CAD build for the part. Positions are in the model's coordinates, mm. A direction names the side the tool comes from. Coordinates: 2 decimals unless noted, no trailing zeros. Loops run counter-clockwise (first coordinate to the right, second up) from the corner with the lowest first, then second, coordinate; pieces in that order, holes last.
1) Saw through at C-C, the plane y = 16.5. Write the cut outline in (x, z), and give its area (3 significant figures).
2) Pin check, flat tips, straight feed: pin 1 Ø0.6 at (x, z) = (4, 5) entering from +Y; pin 2 Ø1.3 at (y, z) = (4, 2.5) entering from -X; pin 3 Ø3 at (x, z) = (10.5, 2) entering from -Y. Stop position of each tip, or through.
3) Two-plate mould, pull along X, no slides. Class faces 4 (the flat face through (18.3, 2, 3)), 5 (the flat face through (0.1, 36, 3)), 6 (the flat face through (14.9, 21, 3)): +X half, -X half, draft (parallel to the pull), parting line (faces both ways), or undercut.
4) Which spindle directions (+Z, -Z, +X, -X, +Y, -Y) get a long thin tool onto all of the face, cutting with end or side? Do faces 1 (the flat face through (7.7, 21, 3)), 2 (the flat face through (15, 32, 4.5)), 3 (the flat face through (11, 18.9, 2)). Say none if no direction does.
5) Saw through at B-B, the plane z = 1.95. Give the number of separate pieces and of enclosed holes in the cut face, and give its area (3 significant figures).
6) Wall check: line 1 along Y through (x, z) = (0.5, 2.1); line 2 along Y through (x, z) = (14, 2); line 3 along X through (y, z) = (19, 2.7). Give the ranges that are in metal, low to high.
7) Saw through at A-A, the plane y = 11. Write the cut outline in (x, z), and give its area (3 significant figures).
```python
from build123d import *

# Parameters (mm, degrees)
SKETCH1_W                      = 22.8
SKETCH1_H                      = 40.7
BOSS_EXTRUDE1_DEPTH            = 1.2
FILLET1_R                      = 2
CUT_EXTRUDE1_REACH             = 45.681
SKETCH4_W                      = 15.4
SKETCH4_H                      = 4.4
CUT_EXTRUDE1_DIRECTION_2_DEPTH = 44.681231668
CUT_EXTRUDE2_REACH             = 45.681
SKETCH5_W                      = 8.4
SKETCH5_H                      = 4
SKETCH6_W                      = 4.6
SKETCH6_H                      = 1
SKETCH6_W_2                    = 1.4
SKETCH6_H_2                    = 2.1
BOSS_EXTRUDE3_DEPTH            = 4.2
SKETCH7_W                      = 1.2
SKETCH7_H                      = 2.8
BOSS_EXTRUDE4_DEPTH            = 4.2
BOSS_EXTRUDE5_DEPTH            = 2
BOSS_EXTRUDE6_DEPTH            = 1.2
SKETCH10_W                     = 2
SKETCH10_H                     = 4
SKETCH10_W_2                   = 4
SKETCH10_H_2                   = 2
CUT_EXTRUDE3_DEPTH             = 0.8
SKETCH11_W                     = 7.2
SKETCH11_H                     = 8
SKETCH11_W_2                   = 4
SKETCH11_H_2                   = 2
SKETCH11_H_3                   = 6.2
SKETCH11_W_3                   = 2
SKETCH11_H_4                   = 4
BOSS_EXTRUDE7_DEPTH            = 3.3
SKETCH12_W                     = 2
SKETCH12_H                     = 5
BOSS_EXTRUDE8_DEPTH            = 3
SKETCH13_W                     = 1.4
SKETCH13_H                     = 14.55
SKETCH13_H_2                   = 8.35
SKETCH13_H_3                   = 12.25
BOSS_EXTRUDE9_DEPTH            = 1.2


with BuildPart() as part:
    # Sketch1 → Boss-Extrude1 (new body)
    with BuildSketch(Plane.XY):
        with Locations((9.2, 18.15)):
            Rectangle(SKETCH1_W, SKETCH1_H)
    extrude(amount=BOSS_EXTRUDE1_DEPTH)

    # Fillet1
    fillet1_edges = [part.edges().sort_by_distance(p)[0] for p in [
        (-2.2, 38.5, 0.6),
        (20.6, 38.5, 0.6),
        (20.6, -2.2, 0.6),
        (-2.2, -2.2, 0.6),
    ]]
    fillet(fillet1_edges, radius=FILLET1_R)

    # Sketch4 → Cut-Extrude1 (cut, up to next)
    with BuildSketch(Plane.XY.offset(1.2), mode=Mode.PRIVATE) as cut_extrude1_sk1:
        with Locations((9.2, 0)):
            Rectangle(SKETCH4_W, SKETCH4_H)
    cut_extrude1_tool1 = extrude(cut_extrude1_sk1.sketch, amount=-CUT_EXTRUDE1_REACH, mode=Mode.PRIVATE) & part.part
    add(cut_extrude1_tool1.solids().sort_by_distance((9.2, 0, 1.2))[0], mode=Mode.SUBTRACT)

    # Sketch4 → Cut-Extrude1 direction 2 (cut)
    with BuildSketch(Plane.XY.offset(1.2)):
        with Locations((9.2, 0)):
            Rectangle(SKETCH4_W, SKETCH4_H)
    extrude(amount=CUT_EXTRUDE1_DIRECTION_2_DEPTH, mode=Mode.SUBTRACT)

    # Sketch5 → Cut-Extrude2 (cut, up to next)
    with BuildSketch(Plane.XY.offset(1.2), mode=Mode.PRIVATE) as cut_extrude2_sk1:
        with Locations((8.8, 4.2)):
            Rectangle(SKETCH5_W, SKETCH5_H)
    cut_extrude2_tool1 = extrude(cut_extrude2_sk1.sketch, amount=-CUT_EXTRUDE2_REACH, mode=Mode.PRIVATE) & part.part
    add(cut_extrude2_tool1.solids().sort_by_distance((8.8, 4.2, 1.2))[0], mode=Mode.SUBTRACT)

    # Sketch6 → Boss-Extrude3 (add)
    with BuildSketch(Plane.XY.offset(1.2)):
        with Locations((16, 35.7)):
            Rectangle(SKETCH6_W, SKETCH6_H)
        with Locations((2.4, 35.7)):
            Rectangle(SKETCH6_W, SKETCH6_H)
        with Locations((0.8, 1.15)):
            Rectangle(SKETCH6_W_2, SKETCH6_H_2)
        with Locations((17.6, 1.15)):
            Rectangle(SKETCH6_W_2, SKETCH6_H_2)
    extrude(amount=BOSS_EXTRUDE3_DEPTH)

    # Sketch7 → Boss-Extrude4 (add)
    with BuildSketch(Plane.XY.offset(1.2)):
        Polygon((0.1, 3.4), (0.1, 2.2), (1.5, 2.2), (4.6, 2.2), (4.6, 3.4), (3.4, 3.4), align=None)
        with Locations((4, 4.8)):
            Rectangle(SKETCH7_W, SKETCH7_H)
    extrude(amount=BOSS_EXTRUDE4_DEPTH)

    # Sketch8 → Boss-Extrude5 (add)
    with BuildSketch(Plane.XY.offset(1.2)):
        Polygon((4.6, 6.2), (13, 6.2), (13, 7.4), (3.4, 7.4), (3.4, 6.2), align=None)
        Polygon((13, 3.4), (14.2, 3.4), (14.2, 7.4), (13, 7.4), (13, 6.2), align=None)
        Polygon((16.9, 2.2), (18.3, 2.2), (18.3, 3.4), (14.2, 3.4), (13, 3.4), (13, 2.2), align=None)
    extrude(amount=BOSS_EXTRUDE5_DEPTH)

    # Sketch9 → Boss-Extrude6 (add)
    with BuildSketch(Plane.XY.offset(3.2)):
        Polygon((13, 7.4), (13, 6.2), (13, 2.2), (16.9, 2.2), (18.3, 2.2), (18.3, 3.4), (14.2, 3.4), (14.2, 7.4), align=None)
    extrude(amount=BOSS_EXTRUDE6_DEPTH)

    # Sketch10 → Cut-Extrude3 (cut)
    with BuildSketch(Plane.XY.offset(1.2)):
        with Locations((16.9, 32.6)):
            Rectangle(SKETCH10_W, SKETCH10_H)
        with Locations((11.3, 22.7)):
            Rectangle(SKETCH10_W_2, SKETCH10_H_2)
        with Locations((11.3, 19.9)):
            Rectangle(SKETCH10_W_2, SKETCH10_H_2)
    extrude(amount=-CUT_EXTRUDE3_DEPTH, mode=Mode.SUBTRACT)

    # Sketch11 → Boss-Extrude7 (add)
    # profile 1 of 2: a face of its own
    with BuildSketch(Plane.XY.offset(1.2)):
        with Locations((11.3, 21.3)):
            Rectangle(SKETCH11_W, SKETCH11_H)
        with Locations((11.3, 19.9)):
            Rectangle(SKETCH11_W_2, SKETCH11_H_2, mode=Mode.SUBTRACT)
        with Locations((11.3, 22.7)):
            Rectangle(SKETCH11_W_2, SKETCH11_H_2, mode=Mode.SUBTRACT)
    # profile 2 of 2: a face of its own
    with BuildSketch(Plane.XY.offset(1.2)):
        with Locations((16.3, 32.1)):
            Rectangle(SKETCH11_W_2, SKETCH11_H_3)
        with Locations((16.9, 32.6)):
            Rectangle(SKETCH11_W_3, SKETCH11_H_4, mode=Mode.SUBTRACT)
    extrude(amount=BOSS_EXTRUDE7_DEPTH)

    # Sketch12 → Boss-Extrude8 (add)
    with BuildSketch(Plane.XY.offset(1.2)):
        with Locations((1.1, 18.15)):
            Rectangle(SKETCH12_W, SKETCH12_H)
        with Locations((17.3, 18.15)):
            Rectangle(SKETCH12_W, SKETCH12_H)
    extrude(amount=BOSS_EXTRUDE8_DEPTH)

    # Sketch13 → Boss-Extrude9 (add)
    with BuildSketch(Plane.XY.offset(1.2)):
        with Locations((1.4, 27.925)):
            Rectangle(SKETCH13_W, SKETCH13_H)
        with Locations((17, 24.825)):
            Rectangle(SKETCH13_W, SKETCH13_H_2)
        with Locations((17, 9.525)):
            Rectangle(SKETCH13_W, SKETCH13_H_3)
        with Locations((1.4, 9.525)):
            Rectangle(SKETCH13_W, SKETCH13_H_3)
    extrude(amount=BOSS_EXTRUDE9_DEPTH)


solid = part.part
```
Data:
1. outline: (-2.2, 0) - (20.6, 0) - (20.6, 1.2) - (18.3, 1.2) - (18.3, 4.2) - (16.3, 4.2) - (16.3, 1.2) - (2.1, 1.2) - (2.1, 4.2) - (0.1, 4.2) - (0.1, 1.2) - (-2.2, 1.2) - close
1. area: 39.4 mm2
2. pin 1: stops at y = 36.2
2. pin 2: stops at x = 0.1
2. pin 3: stops at y = 6.2
3. face 4: +X half
3. face 5: -X half
3. face 6: undercut
4. face 1: +Z, +Y
4. face 2: +Z, +X, -X
4. face 3: +Z
5. separate pieces: 2
5. enclosed holes: 3
5. area: 191 mm2
6. line 1: y = 0.1 to 3.4, 15.65 to 20.65, 35.2 to 36.2
6. line 2: y = 2.2 to 7.4, 17.3 to 25.3, 35.2 to 36.2
6. line 3: x = 0.1 to 2.1, 7.7 to 9.3, 13.3 to 14.9, 16.3 to 18.3
7. outline: (-2.2, 0) - (20.6, 0) - (20.6, 1.2) - (17.7, 1.2) - (17.7, 2.4) - (16.3, 2.4) - (16.3, 1.2) - (2.1, 1.2) - (2.1, 2.4) - (0.7, 2.4) - (0.7, 1.2) - (-2.2, 1.2) - close
7. area: 30.7 mm2
